```python
from build123d import *

# Parameters (mm, degrees)
SKICA1_W                 = 110
SKICA1_H                 = 50
SKICA1_W_2               = 82
SKICA1_H_2               = 46
P_IDAT_VYSUNUT_M1_DEPTH  = 2
SKICA2_R                 = 1.4
P_IDAT_VYSUNUT_M2_DEPTH  = 2
ZAOBLIT1_R               = 5
SKICA3_R                 = 1.4
ODEBRAT_VYSUNUT_M1_DEPTH = 2
P_IDAT_START             = 3
SKICA4_R                 = 1.4
P_IDAT_VYSUNUT_M3_DEPTH  = 3
SKICA5_R                 = 1.4
P_IDAT_VYSUNUT_M5_DEPTH  = 2.2
SKICA6_R                 = 1.4
ODEBRAT_VYSUNUT_M2_DEPTH = 2
P_IDAT_VYSUNUT_M6_REACH  = 122.868
SKICA8_W                 = 3
SKICA8_H                 = 19.8
ZKOSEN_1_SIZE            = 3
SKICA9_W                 = 68
SKICA9_H                 = 3.5
SKICA9_W_2               = 3.5
SKICA9_H_2               = 24
P_IDAT_VYSUNUT_M7_DEPTH  = 2


with BuildPart() as part:
    # Skica1 → Přidat vysunutím1 (new body)
    with BuildSketch(Plane.XY):
        with Locations((55, 25)):
            Rectangle(SKICA1_W, SKICA1_H)
        with Locations((43, 25)):
            Rectangle(SKICA1_W_2, SKICA1_H_2, mode=Mode.SUBTRACT)
    extrude(amount=P_IDAT_VYSUNUT_M1_DEPTH)

    # Skica2 → Přidat vysunutím2 (add)
    # profile 1 of 4: a face of its own
    with BuildSketch(Plane(origin=(0, 0, 0), x_dir=(-1, 0, 0), z_dir=(0, 0, -1))):
        with BuildLine():
            Line((-77, 42), (-77, 48))
            Line((-77, 48), (-84, 48))
            Line((-84, 48), (-84, 38.5))
            Line((-84, 38.5), (-80.5, 38.5))
            ThreePointArc((-80.5, 38.5), (-78.025126266, 39.525126266), (-77, 42))
        make_face()
        with Locations((-80.5, 42)):
            Circle(SKICA2_R, mode=Mode.SUBTRACT)
    # profile 2 of 4: a face of its own
    with BuildSketch(Plane(origin=(0, 0, 0), x_dir=(-1, 0, 0), z_dir=(0, 0, -1))):
        with BuildLine():
            Line((-9, 42), (-9, 48))
            Line((-9, 48), (-2, 48))
            Line((-2, 48), (-2, 38.5))
            Line((-2, 38.5), (-5.5, 38.5))
            ThreePointArc((-5.5, 38.5), (-7.974873734, 39.525126266), (-9, 42))
        make_face()
        with Locations((-5.5, 42)):
            Circle(SKICA2_R, mode=Mode.SUBTRACT)
    # profile 3 of 4: a face of its own
    with BuildSketch(Plane(origin=(0, 0, 0), x_dir=(-1, 0, 0), z_dir=(0, 0, -1))):
        with BuildLine():
            Line((-80.5, 14.5), (-84, 14.5))
            Line((-84, 14.5), (-84, 2))
            Line((-84, 2), (-77, 2))
            Line((-77, 2), (-77, 11))
            ThreePointArc((-77, 11), (-78.025126266, 13.474873734), (-80.5, 14.5))
        make_face()
        with Locations((-80.5, 4.8)):
            Circle(SKICA2_R, mode=Mode.SUBTRACT)
    # profile 4 of 4: a face of its own
    with BuildSketch(Plane(origin=(0, 0, 0), x_dir=(-1, 0, 0), z_dir=(0, 0, -1))):
        with BuildLine():
            Line((-5.5, 14.5), (-2, 14.5))
            Line((-2, 14.5), (-2, 2))
            Line((-2, 2), (-9, 2))
            Line((-9, 2), (-9, 11))
            ThreePointArc((-9, 11), (-7.974873734, 13.474873734), (-5.5, 14.5))
        make_face()
        with Locations((-5.5, 4.8)):
            Circle(SKICA2_R, mode=Mode.SUBTRACT)
    extrude(amount=-P_IDAT_VYSUNUT_M2_DEPTH)

    # Zaoblit1
    zaoblit1_edges = [part.edges().sort_by_distance(p)[0] for p in [
        (0, 50, 1),
        (110, 50, 1),
        (110, 0, 1),
        (0, 0, 1),
    ]]
    fillet(zaoblit1_edges, radius=ZAOBLIT1_R)

    # Skica3 → Odebrat vysunutím1 (cut)
    with BuildSketch(Plane.XY.offset(2)):
        with Locations((101.05, 29.1)):
            Circle(SKICA3_R)
        with Locations((101.05, 15.3)):
            Circle(SKICA3_R)
    extrude(amount=-ODEBRAT_VYSUNUT_M1_DEPTH, mode=Mode.SUBTRACT)

    # Skica4 → Přidat vysunutím3 (add)
    with BuildSketch(Plane.XY.offset(2).offset(P_IDAT_START)):
        with BuildLine():
            Line((104.05, 29.1), (104.05, 15.3))
            ThreePointArc((104.05, 15.3), (101.05, 12.3), (98.05, 15.3))
            Line((98.05, 15.3), (98.05, 29.1))
            ThreePointArc((98.05, 29.1), (101.05, 32.1), (104.05, 29.1))
        make_face()
        with Locations((101.05, 15.3)):
            Circle(SKICA4_R, mode=Mode.SUBTRACT)
        with Locations((101.05, 29.1)):
            Circle(SKICA4_R, mode=Mode.SUBTRACT)
    extrude(amount=-P_IDAT_VYSUNUT_M3_DEPTH)

    # Skica5 → Přidat vysunutím5 (add)
    # profile 1 of 4: a face of its own
    with BuildSketch(Plane.XY.offset(2)):
        with BuildLine():
            Line((2, 45), (2, 38.5))
            Line((2, 38.5), (5.5, 38.5))
            ThreePointArc((5.5, 38.5), (7.974873734, 39.525126266), (9, 42))
            Line((9, 42), (9, 48))
            Line((9, 48), (5, 48))
            ThreePointArc((5, 48), (2.878679656, 47.121320344), (2, 45))
        make_face()
        with Locations(Location((5.5, 42, 0), (0, 0, 180))):
            Circle(SKICA5_R, mode=Mode.SUBTRACT)
    # profile 2 of 4: a face of its own
    with BuildSketch(Plane.XY.offset(2)):
        with BuildLine():
            Line((5.5, 14.5), (2, 14.5))
            Line((2, 14.5), (2, 5))
            ThreePointArc((2, 5), (2.878679656, 2.878679656), (5, 2))
            Line((5, 2), (9, 2))
            Line((9, 2), (9, 11))
            ThreePointArc((9, 11), (7.974873734, 13.474873734), (5.5, 14.5))
        make_face()
        with Locations(Location((5.5, 4.8, 0), (0, 0, 180))):
            Circle(SKICA5_R, mode=Mode.SUBTRACT)
    # profile 3 of 4: a face of its own
    with BuildSketch(Plane.XY.offset(2)):
        with BuildLine():
            Line((84, 48), (77, 48))
            Line((77, 48), (77, 42))
            ThreePointArc((77, 42), (78.025126266, 39.525126266), (80.5, 38.5))
            Line((80.5, 38.5), (84, 38.5))
            Line((84, 38.5), (84, 48))
        make_face()
        with Locations(Location((80.5, 42, 0), (0, 0, 180))):
            Circle(SKICA5_R, mode=Mode.SUBTRACT)
    # profile 4 of 4: a face of its own
    with BuildSketch(Plane.XY.offset(2)):
        with BuildLine():
            Line((77, 11), (77, 2))
            Line((77, 2), (84, 2))
            Line((84, 2), (84, 14.5))
            Line((84, 14.5), (80.5, 14.5))
            ThreePointArc((80.5, 14.5), (78.025126266, 13.474873734), (77, 11))
        make_face()
        with Locations(Location((80.5, 4.8, 0), (0, 0, 180))):
            Circle(SKICA5_R, mode=Mode.SUBTRACT)
    extrude(amount=P_IDAT_VYSUNUT_M5_DEPTH)

    # Skica6 → Odebrat vysunutím2 (cut)
    with BuildSketch(Plane(origin=(0, 0, 0), x_dir=(-1, 0, 0), z_dir=(0, 0, -1))):
        with Locations((-104.5, 42)):
            Circle(SKICA6_R)
        with Locations((-104.5, 4.8)):
            Circle(SKICA6_R)
    extrude(amount=-ODEBRAT_VYSUNUT_M2_DEPTH, mode=Mode.SUBTRACT)

    # Přidat vysunutím6: up to this face of the body (flat: up to its plane)
    p_idat_vysunut_m6_end = Plane(part.part.faces().sort_by_distance((101.05, 22.2, 5))[0])
    # Skica8 → Přidat vysunutím6 (add, up to the picked face)
    with BuildSketch(Plane.XY.offset(2), mode=Mode.PRIVATE) as p_idat_vysunut_m6_sk1:
        with Locations((85.5, 22.2)):
            Rectangle(SKICA8_W, SKICA8_H)
    p_idat_vysunut_m6_tool1 = split(extrude(p_idat_vysunut_m6_sk1.sketch, amount=P_IDAT_VYSUNUT_M6_REACH, mode=Mode.PRIVATE), bisect_by=p_idat_vysunut_m6_end, keep=Keep.BOTH, mode=Mode.PRIVATE)
    add(p_idat_vysunut_m6_tool1.solids().sort_by(Axis((85.5, 22.2, 2), (0, 0, 1)))[0])

    # Zkosení1
    zkosen_1_edges = [part.edges().sort_by_distance(p)[0] for p in [
        (87, 22.2, 2),
    ]]
    chamfer(zkosen_1_edges, length=ZKOSEN_1_SIZE - 0.0001)  # a hair under: the kernel refuses the full size

    # Skica9 → Přidat vysunutím7 (add)
    with BuildSketch(Plane(origin=(0, 0, 0), x_dir=(-1, 0, 0), z_dir=(0, 0, -1))):
        with Locations((-43, 3.75)):
            Rectangle(SKICA9_W, SKICA9_H)
        with Locations((-43, 46.25)):
            Rectangle(SKICA9_W, SKICA9_H)
        with Locations((-3.75, 26.5)):
            Rectangle(SKICA9_W_2, SKICA9_H_2)
    extrude(amount=-P_IDAT_VYSUNUT_M7_DEPTH)


solid = part.part
```
The model under review builds one solid part; all positions refer to its coordinate system, in mm. A direction names the side the tool comes from. Give positions to 0.01 mm unless a question says otherwise; leave off trailing zeros. Loops run counter-clockwise (first coordinate to the right, second up) from the corner with the lowest first, then second, coordinate; pieces in that order, holes last. Notation, with made-up numbers: (56, 62.25) - (98, 62.25) arc R18 ccw to (98, 92.25) - close; hole circle Ø11 at (-21.5, 49.25). An arc over 180 degrees is marked (long way). Answer as a JSON object with one key per item and string values.
Q1. Insertion check: pin 1 (2.5 mm diameter, centred on x = 80.5, y = 42, fed in from -Z); pin 2 (0.7 mm diameter, centred on x = 79, z = 3, fed in from +Y); pin 3 (2.5 mm diameter, centred on y = 21.5, z = 4, fed in from -X); pin 4 (5.5 mm diameter, centred on x = 80, y = 42.5, fed in from +Z). Each pin has a flat end and moves straight along its axis. Give the tip position at first contact, or say it passes through.
Worked out:
{"pin 1": "passes through", "pin 2": "stops at y = 48", "pin 3": "stops at x = 84", "pin 4": "stops at z = 4.2"}
Q2. Add section D-D on x = 88. State the section outline as (y, z) points, plus the area to 3 significant figures.
Worked out:
{"outline": "(0, 0) - (50, 0) - (50, 2) - (32.1, 2) - (32.1, 4) - (12.3, 4) - (12.3, 2) - (0, 2) - close", "area": "140 mm^2"}
Q3. For faces 1 (the flat face through (2, 42, 3)), 2 (the flat face through (80, 2, 3)), 3 (the flat face through (5.5, 26, 1)), list the 3-axis set-ups (+Z, -Z, +X, -X, +Y, -Y) from which the entire face can be reached by the end or side of a thin tool; tool diameter is ignored.
Worked out:
{"face 1": "+Z, -X, +Y, -Y", "face 2": "+Z, +X, -X, -Y", "face 3": "+Z, -Z"}
Q4. To check wall thickness, follow line 1 along Y through (x, z) = (80.5, 1.6); line 2 along X through (y, z) = (4.8, 3); line 3 along Y through (x, z) = (104.5, 1.5). State the ranges of each line that lie inside material, in increasing order.
Worked out:
{"line 1": "y = 0 to 3.4, 6.2 to 14.5, 38.5 to 40.6, 43.4 to 50", "line 2": "x = 2.01 to 4.1, 6.9 to 9, 77 to 79.1, 81.9 to 84", "line 3": "y = 0 to 3.4, 6.2 to 40.6, 43.4 to 50"}
Q5. Mouldability with a two-part tool opening along Y and no side actions: class faces 4 (the flat face through (43, 5.5, 1)), 5 (the flat face through (84, 43, 3)), 6 (the cylindrical face through (2.9, 47.14, 3.08)) as +Y half, -Y half, draft (parallel to the pull), parting line (faces both ways), or undercut.
Worked out:
{"face 4": "undercut", "face 5": "draft", "face 6": "+Y half"}
Q6. Add section B-B on x = 101.05. State the section outline as (y, z) points, plus the area to 3 significant figures.
Worked out:
{"outline": "(0, 0) - (13.9, 0) - (13.9, 5) - (12.3, 5) - (12.3, 2) - (0, 2) - close; (16.7, 0) - (27.7, 0) - (27.7, 5) - (16.7, 5) - close; (30.5, 0) - (50, 0) - (50, 2) - (32.1, 2) - (32.1, 5) - (30.5, 5) - close", "area": "131 mm^2"}
Q7. Add section C-C on y = 39.5. State the section outline as (x, z) points.
Worked out:
{"outline": "(0, 0) - (7.95, 0) - (7.95, 4.2) - (2, 4.2) - (2, 2) - (0, 2) - close; (78.05, 0) - (110, 0) - (110, 2) - (84, 2) - (84, 4.2) - (78.05, 4.2) - close"}
Q8. Add section A-A on x = 60.5. State the section outline as (y, z) points, plus the area to 3 significant figures.
Worked out:
{"outline": "(0, 0) - (5.5, 0) - (5.5, 2) - (0, 2) - close; (44.5, 0) - (50, 0) - (50, 2) - (44.5, 2) - close", "area": "22.0 mm^2"}
